Autodesk Inventor part; units mm, degrees
ref_plane "XY Plane" through (0, 0, 0) normal (0, 0, 1) x (1, 0, 0)
ref_plane "Work Plane1" through (0, 0, 36.5) normal (0, 0, 1) x (1, 0, 0)
sketch "Sketch1" plane through (0, 0, 0) normal (0, 0, 1) x (1, 0, 0)
  circle A0 centre (0, 0) radius 17.5
  circle A1 centre (0, 0) radius 21
  dimension "d1" = 42
  dimension "d2" = 35
extrude "Extrusion1" add sketch "Sketch1" along normal blind 52 contours A0 | A1
sketch "Sketch2" plane through (0, 0, 0) normal (0, 1, 0) x (-1, 0, 0)
  circle A0 centre (0, 0) radius 17.5
  circle A1 centre (0, 0) radius 21
  dimension "d5" = 35
  dimension "d6" = 42
extrude "Extrusion2" add sketch "Sketch2" along normal mid plane 56 contours A0 | A1
extrude "Extrusion3" cut sketch "Sketch2" against normal up to surface (56 mm away) from surface at 28 contours A0
extrude "Extrusion4" cut sketch "Sketch1" along normal up to surface (52 mm away) contours A0
fillet "Fillet1" radius 5 2 edges at (0, 21, 21) (0, -21, 21)
hole "Hole1" at (0, 0, 0) direction (-1, 0, 0) diameter 6.647 end through all
ref_plane "Work Plane1" through (0, 0, 36.5) normal (0, 0, 1) x (1, 0, 0)
hole "Hole2" at (0, 0, 36.5) direction (0, -1, 0) diameter 6.647 end through all
fillet "Fillet2" radius 2 3 edges at (21, 28, 0) (-21, 0, 52) (21, -28, 0)
equation "\"d5\" = d2"
equation "\"d6\" = d1"
equation "\"d23\" = -0.5 * d3 + 0.25 * d1"
properties part number "L10-6" material "Aluminium Cast"
CAD build for the part. Positions are in the model's coordinates, mm. A direction names the side the tool comes from. Round coordinates to 2 decimals unless told otherwise and drop trailing zeros. Write each loop counter-clockwise with the first axis right and the second up, starting at its lowest first coordinate (ties: lowest second). Pieces come first, ordered by that corner, then holes. Notation, with made-up numbers: M -7.5,13 L 40.5,13 A11 cw 40.5,34 Z; hole C -25.75,21.25 d11. An arc over 180 degrees is marked long. Put each result on its own line as item: value. Start each with the question number.
1) 3-axis set-ups, long thin cutter, end or side, ignore diameter. For faces 1 (the cylindrical face through (8.075, 15.526, 31.414)), 2 (the cylindrical face through (-0.15, -19.12, 33.18)), 3 (the cylindrical face through (4.55, 0.36, -20.5)): which of +Z, -Z, +X, -X, +Y, -Y reach the whole face in a straight line?
2) Saw through at B-B, the plane x = 9.5. Count the separate pieces of the cut face and the enclosed holes in it, and give its area (3 significant figures).
3) Saw through at A-A, the plane z = 29. Write the cut outline in (x, y), and give its area (3 significant figures).
4) Pull direction Y, two halves, no side cores. Call faces 4 (the flat face through (-6, 28, -17)), 5 (the cylindrical face through (9.69, 18.63, 30.21)), 6 (the cylindrical face through (-19.118, -2.246, 2.45)): pulls with the +Y half, pulls with the -Y half, needs draft (parallel to the pull), parting line crosses it, or undercut.
5) Drill centre lines: probe 1 along Y at (x, z) = (-19.1, 0); probe 2 along X at (y, z) = (0, 23); probe 3 along Y at (x, z) = (0, 19). Where is each one in solid material? Low to high. Write a range as [from, to].
6) Pin check, flat tips, straight feed: pin 1 Ø3 at (y, z) = (12.5, 3.5) entering from +X; pin 2 Ø8 at (y, z) = (-12, 30) entering from +X; pin 3 Ø5 at (x, z) = (15.5, 35.5) entering from +Y. Stop position of each tip, or through.
Resolved:
1. face 1: +Z
1. face 2: -Y
1. face 3: none
2. separate pieces: 3
2. enclosed holes: 0
2. area: 603 mm²
3. outline: C 0,0 d42; hole C 0,0 d35
3. area: 423 mm²
4. face 4: pulls with the +Y half
4. face 5: parting line crosses it
4. face 6: undercut
5. probe 1: [-28, -3.32], [3.32, 28]
5. probe 2: [-21, -17.5], [17.5, 21]
5. probe 3: [-28, -17.5], [17.5, 28]
6. pin 1: x = 20.9
6. pin 2: x = 19.42
6. pin 3: y = 16.49
